Input: part model. Units: mm. Frame: model coordinates. Round coordinates to 2 decimals unless told otherwise and drop trailing zeros. Write each loop counter-clockwise with the first axis right and the second up, starting at its lowest first coordinate (ties: lowest second). Pieces come first, ordered by that corner, then holes. Notation, with made-up numbers: (-24.5, 76) - (28.5, 76) arc R35 cw to (28.5, 110) - close; hole circle Ø10 at (9.5, 12). An arc over 180 degrees is marked (long way). Use one line per item in the form item = value.
```python
from build123d import *

# Parameters (mm, degrees)
SKETCH1_W           = 135
SKETCH1_H           = 45
BOSS_EXTRUDE1_DEPTH = 5
CUT_EXTRUDE2_REACH  = 73.327
SKETCH3_R           = 2.5
SKETCH4_R           = 6
SKETCH4_R_2         = 1.6
CUT_EXTRUDE3_DEPTH  = 72.326713088


with BuildPart() as part:
    # Sketch1 → Boss-Extrude1 (new body)
    with BuildSketch(Plane(origin=(0, 0, 0), x_dir=(1, 0, 0), z_dir=(0, 1, 0))):
        Rectangle(SKETCH1_W, SKETCH1_H)
    extrude(amount=BOSS_EXTRUDE1_DEPTH)

    # Sketch3 → Cut-Extrude2 (cut, up to next)
    with BuildSketch(Plane.XZ, mode=Mode.PRIVATE) as cut_extrude2_sk1:
        with Locations(Location((-36.498729637, -5.198729637, 0), (0, 0, 270))):
            Circle(SKETCH3_R)
    cut_extrude2_tool1 = extrude(cut_extrude2_sk1.sketch, amount=-CUT_EXTRUDE2_REACH, mode=Mode.PRIVATE) & part.part
    # Sketch3 → Cut-Extrude2 (cut, up to next)
    with BuildSketch(Plane.XZ, mode=Mode.PRIVATE) as cut_extrude2_sk2:
        with Locations(Location((-6.496188911, -5.198729637, 0), (0, 0, 270))):
            Circle(SKETCH3_R)
    cut_extrude2_tool2 = extrude(cut_extrude2_sk2.sketch, amount=-CUT_EXTRUDE2_REACH, mode=Mode.PRIVATE) & part.part
    add(cut_extrude2_tool1.solids().sort_by_distance((-36.49873, 0, -5.19873))[0], mode=Mode.SUBTRACT)
    add(cut_extrude2_tool2.solids().sort_by_distance((-6.496189, 0, -5.19873))[0], mode=Mode.SUBTRACT)

    # Sketch4 → Cut-Extrude3 (cut, through all)
    with BuildSketch(Plane.XZ):
        with Locations(Location((44.5, 0.002540726, 0), (0, 0, 270))):
            Circle(SKETCH4_R)
        with Locations(Location((60, 15.502540726, 0), (0, 0, 270))):
            Circle(SKETCH4_R_2)
        with Locations(Location((29, 15.502540726, 0), (0, 0, 270))):
            Circle(SKETCH4_R_2)
        with Locations(Location((29, -15.497459274, 0), (0, 0, 270))):
            Circle(SKETCH4_R_2)
        with Locations(Location((60, -15.497459274, 0), (0, 0, 270))):
            Circle(SKETCH4_R_2)
    extrude(amount=-CUT_EXTRUDE3_DEPTH, mode=Mode.SUBTRACT)


solid = part.part
```
(1) Cut plane D-D on y = 3.45. Output: boundary loops of the cut face in (x, z), then the cut area to 3 significant figures.
Derived:
outline = (-67.5, -22.5) - (67.5, -22.5) - (67.5, 22.5) - (-67.5, 22.5) - close; hole circle Ø5 at (-36.5, -5.2); hole circle Ø5 at (-6.5, -5.2); hole circle Ø3.2 at (29, -15.5); hole circle Ø3.2 at (29, 15.5); hole circle Ø12 at (44.5, 0); hole circle Ø3.2 at (60, -15.5); hole circle Ø3.2 at (60, 15.5)
area = 5,890 mm^2
(2) Material intervals for L1, parallel to X at y = 3.4, z = 14.5; L2, parallel to X at y = 3.8, z = 15; L3, parallel to Z at x = 28, y = 3.9, sorted ascending.
Derived:
L1 = -67.5 to 27.75, 30.25 to 58.75, 61.25 to 67.5
L2 = -67.5 to 27.48, 30.52 to 58.48, 61.52 to 67.5
L3 = -22.5 to -16.75, -14.25 to 14.25, 16.75 to 22.5
(3) Draft query along X for faces 1 (the face through (-1, 5, 0)), 2 (the face through (67.5, 2, 0)), 3 (the face through (-38.94, 2.46, -4.66)). Return one class per face: released by +X, released by -X, zero draft, split by the parting line, or undercut.
Derived:
face_1 = zero draft
face_2 = released by +X
face_3 = undercut
(4) Cut plane A-A on x = 29. Output: boundary loops of the cut face in (y, z), then the cut area to 3 significant figures.
Derived:
outline = (0, -22.5) - (5, -22.5) - (5, -17.1) - (0, -17.1) - close; (0, -13.9) - (5, -13.9) - (5, 13.9) - (0, 13.9) - close; (0, 17.1) - (5, 17.1) - (5, 22.5) - (0, 22.5) - close
area = 193 mm^2
(5) Cut plane C-C on z = 0. Output: boundary loops of the cut face in (x, y), then the cut area to 3 significant figures.
Derived:
outline = (-67.5, 0) - (38.5, 0) - (38.5, 5) - (-67.5, 5) - close; (50.5, 0) - (67.5, 0) - (67.5, 5) - (50.5, 5) - close
area = 615 mm^2
(6) Cut plane B-B on x = 44.5. Output: boundary loops of the cut face in (y, z), then the cut area to 3 significant figures.
Derived:
outline = (0, -22.5) - (5, -22.5) - (5, -6) - (0, -6) - close; (0, 6) - (5, 6) - (5, 22.5) - (0, 22.5) - close
area = 165 mm^2
(7) First-contact query: pin 1 Ø2.5 at (x, z) = (29, -15.5) entering from +Y; pin 2 Ø5 at (x, z) = (60, -15.5) entering from +Y. Flat tips, straight axial feed; report the tip coordinate or a pass-through.
Derived:
pin_1 = through
pin_2 = 5
